```python
from build123d import *

# Parameters (mm, degrees)
BOSS_EXTRUDE1_DEPTH = 0.254
SKETCH2_R           = 4.699
CUT_EXTRUDE1_DEPTH  = 1.254
SKETCH3_W           = 2.54
SKETCH3_H           = 0.635
CUT_EXTRUDE2_DEPTH  = 1.254
SKETCH5_OUTSIDE_W   = 121.447
SKETCH5_OUTSIDE_H   = 109.618
CUT_EXTRUDE5_DEPTH  = 1.254


with BuildPart() as part:
    # Sketch1 → Boss-Extrude1 (new body)
    with BuildSketch(Plane.XY):
        with BuildLine():
            Line((67.21146711, 76.191723231), (8.696654013, 17.676910134))
            Line((8.696654013, 17.676910134), (7.228954972, 14.133571205))
            ThreePointArc((7.228954972, 14.133571205), (14.666587579, 6.075099489), (15.105587123, -4.88230096))
            Line((15.105587123, -4.88230096), (18.648926052, -6.35))
            Line((18.648926052, -6.35), (101.401368334, -6.35))
            ThreePointArc((101.401368334, -6.35), (93.866160503, 38.880636728), (67.21146711, 76.191723231))
        make_face()
        with BuildLine():
            Line((88.672924278, 6.35), (27.86051193, 6.35))
            ThreePointArc((27.86051193, 6.35), (26.399857642, 10.93517908), (24.190484974, 15.210228852))
            Line((24.190484974, 15.210228852), (67.191354125, 58.211098004))
            ThreePointArc((67.191354125, 58.211098004), (82.13289044, 34.020557137), (88.672924278, 6.35))
        make_face(mode=Mode.SUBTRACT)
    extrude(amount=BOSS_EXTRUDE1_DEPTH)

    # Sketch2 → Cut-Extrude1 (cut, through all)
    with BuildSketch(Plane.XY.offset(0.254)):
        with Locations((22.225, 0)):
            Circle(SKETCH2_R)
        with Locations((36.195, 0)):
            Circle(SKETCH2_R)
        with Locations((61.722, 0)):
            Circle(SKETCH2_R)
        with Locations((75.692, 0)):
            Circle(SKETCH2_R)
        with Locations((95.25, 0)):
            Circle(SKETCH2_R)
        with Locations((15.715448212, 15.715448212)):
            Circle(SKETCH2_R)
        with Locations((25.593729945, 25.593729945)):
            Circle(SKETCH2_R)
        with Locations((43.644044748, 43.644044748)):
            Circle(SKETCH2_R)
        with Locations((53.522326482, 53.522326482)):
            Circle(SKETCH2_R)
        with Locations((92.004434954, 24.652514046)):
            Circle(SKETCH2_R)
        with Locations((82.48891971, 47.625)):
            Circle(SKETCH2_R)
        with Locations((67.351920908, 67.351920908)):
            Circle(SKETCH2_R)
    extrude(amount=-CUT_EXTRUDE1_DEPTH, mode=Mode.SUBTRACT)

    # Sketch3 → Cut-Extrude2 (cut, through all)
    with BuildSketch(Plane.XY.offset(0.254)):
        Polygon((15.266435406, 24.246691527), (17.06248663, 26.042742751), (17.511499436, 25.593729945), (15.715448212, 23.797678721), align=None)
        Polygon((44.991083167, 53.971339288), (43.195031942, 52.175288063), (43.644044748, 51.726275257), (45.440095973, 53.522326482), align=None)
        with Locations((29.21, -6.0325)):
            Rectangle(SKETCH3_W, SKETCH3_H)
        with Locations((68.707, -6.0325)):
            Rectangle(SKETCH3_W, SKETCH3_H)
        Polygon((29.230733674, 38.210989795), (31.026784898, 40.007041019), (31.475797704, 39.558028213), (29.67974648, 37.761976989), align=None)
        Polygon((56.845021246, 65.825277367), (55.048970022, 64.029226143), (55.497982828, 63.580213337), (57.294034052, 65.376264561), align=None)
        with Locations((48.9585, -6.0325)):
            Rectangle(SKETCH3_W, SKETCH3_H)
        with Locations((85.471, -6.0325)):
            Rectangle(SKETCH3_W, SKETCH3_H)
        Polygon((99.935462164, 14.437711971), (100.266998693, 11.919442024), (101.526133667, 12.085210288), (101.194597138, 14.603480236), align=None)
        Polygon((93.765504959, 37.464305742), (94.938831965, 37.950313702), (93.966816047, 40.296967714), (92.793489041, 39.810959755), align=None)
        Polygon((79.327792988, 62.471156422), (80.874047017, 60.456038938), (81.88160576, 61.229165953), (80.33535173, 63.244283437), align=None)
        Polygon((13.593916116, 7.005422516), (14.565932035, 4.658768503), (15.739259041, 5.144776462), (14.767243123, 7.491430475), align=None)
    extrude(amount=-CUT_EXTRUDE2_DEPTH, mode=Mode.SUBTRACT)

    # Sketch5 outside → Cut-Extrude5 (cut, through all)
    with BuildSketch(Plane.XY.offset(0.254)):
        with Locations((54.4145, 34.921)):
            Rectangle(SKETCH5_OUTSIDE_W, SKETCH5_OUTSIDE_H)
        Polygon((11.513421912, 3.394377411), (27.94, 10.198488838), (27.94, -7.62), (11.513421912, -7.62), align=None, mode=Mode.SUBTRACT)
    extrude(amount=-CUT_EXTRUDE5_DEPTH, mode=Mode.SUBTRACT)


solid = part.part
```
The listing builds one solid part. Answer for the finished solid, in the listing's coordinates (mm). Coordinates: 2 decimals unless noted, no trailing zeros. Write each loop counter-clockwise with the first axis right and the second up, starting at its lowest first coordinate (ties: lowest second). Pieces come first, ordered by that corner, then holes. Notation, with made-up numbers: (-9.75, 39.5) - (43.25, 39.5) arc R17 ccw to (43.25, 55.5) - close; hole circle Ø3 at (15.5, 0.5). An arc over 180 degrees is marked (long way). Return JSON: item names as keys, results as strings. Group by question number.
Q1. Find the intervals of material crossed by line 1 along X through (y, z) = (2, 0.2); line 2 along X through (y, z) = (-2.75, 0.1) (3 decimals); line 3 along Y through (x, z) = (26.5, 0.2), in increasing order. Write a range as [from, to].
Q2. The part is cut by section A-A on z = 0.15. Write down the section's boundary in (x, y) (3 decimals).
Q3. The part is cut by section B-B on y = 0. Write down the section's boundary in (x, z) (3 decimals).
Q4. A flat-ended cylindrical pin translates along its axis: pin 1 Ø2 at (x, y) = (18, 2.5) entering from -Z. Find the tip coordinate at first contact, or state that the pin passes through.
Q5. The part is cut by section C-C on x = 24.25. Write down the section's boundary in (y, z), and give its area (3 significant figures).
Evaluation:
{
 "1": {"line 1": "x = [15.75, 17.97], [26.48, 27.94]", "line 2": "x = [15.635, 18.415], [26.035, 27.94]", "line 3": "y = [-6.35, -1.95], [1.95, 9.6]"},
 "2": {"outline": "(15.106, -4.882) - (18.649, -6.35) - (27.94, -6.35) - (27.94, 6.35) - (27.861, 6.35) arc R28.575 ccw to (26.86, 9.751) - (15.106, 4.882) arc R15.875 cw to start; hole circle Ø9.398 at (22.225, 0)"},
 "3": {"outline": "(15.875, 0) - (17.526, 0) - (17.526, 0.254) - (15.875, 0.254) - close; (26.924, 0) - (27.94, 0) - (27.94, 0.254) - (26.924, 0.254) - close"},
 "4": {"pin 1": "stops at z = 0"},
 "5": {"outline": "(-6.35, 0) - (-4.24, 0) - (-4.24, 0.25) - (-6.35, 0.25) - close; (4.24, 0) - (8.67, 0) - (8.67, 0.25) - (4.24, 0.25) - close", "area": "1.66 mm2"}
}
